Autodesk Inventor part; units mm, degrees
ref_plane "YZ Plane" through (0, 0, 0) normal (1, 0, 0) x (0, 1, 0)
ref_plane "XZ Plane" through (0, 0, 0) normal (0, 1, 0) x (-1, 0, 0)
ref_plane "XY Plane" through (0, 0, 0) normal (0, 0, 1) x (1, 0, 0)
sketch "Sketch1" plane through (0, 0, 0) normal (0, 1, 0) x (-1, 0, 0)
  line L0 (-60, 105) -> (60, 105)
  line L1 (60, 105) -> (60, 90)
  line L2 (60, -105) -> (-60, -105)
  line L3 (-60, -105) -> (-60, -90)
  line L4 (-60, 105) -> (60, -105) construction
  line L5 (60, 105) -> (-60, -105) construction
  line L6 (60, 90) -> (-60, 90)
  line L7 (60, -90) -> (-60, -90)
  line L8 (60, 90) -> (60, -90)
  line L9 (60, -90) -> (60, -105)
  line L10 (-60, -90) -> (-60, 90)
  line L11 (-60, 90) -> (-60, 105)
  line L12 (84, 0) -> (-84, 0)
  line L13 (0, -147) -> (0, 147)
  point P0 (0, 0)
  dimension "d0" = 180
  dimension "d1" = 15
  dimension "d2" = 120
extrude "Plate1" add sketch "Sketch1" along normal blind 5 contours L6 L13 L12 L10 | L6 L8 L12 L13 | L12 L13 L7 L10 | L12 L8 L7 L13
sketch "Sketch2" plane through (-60, 5, 85) normal (0, 0, 1) x (1, 0, 0)
  line L0 (120, 0) -> (0, 0)
  line L1 (0, 0) -> (0, -15)
  line L2 (0, -15) -> (120, -15)
  line L3 (120, -15) -> (120, 0)
edge flange "Flange1" height 15 angle 90 thickness 5 bend radius 5 thickness toward (0, 0, 1) relief tear relief width 5 relief depth 2.5 corner gap 5 corner form 0 edges at (0, 0, 90) (0, 0, -90) wall of the first edge with corners at (60, 5, 85) (-60, 5, 85) (-60, -10, 85) (60, -10, 85)
bend "Bend1"
corner "Corner1"
sketch "Sketch3" plane through (0, 0, 0) normal (0, -1, 0) x (1, 0, 0)
  circle A0 centre (-16.2613, 28.9263) radius 2.75
  circle A1 centre (38.7387, 28.9263) radius 2.75
  circle A2 centre (-16.2613, -31.0737) radius 2.75
  circle A3 centre (38.7387, -31.0737) radius 2.75
  point P0 (0, 0)
extrude "Extrusion1" cut sketch "Sketch3" against normal through all
equation "\"d3\" = Thickness"
equation "\"d4\" = BendReliefWidth"
equation "\"d5\" = BendReliefDepth"
equation "\"d6\" = MinimumRemnant"
equation "\"d7\" = TransitionRadius"
equation "\"d10\" = BendRadius"
equation "\"d11\" = CornerReliefSize"
equation "\"d12\" = GapSize"
equation "\"d13\" = JacobiRadiusSize"
equation "\"BendRadius\" = Thickness"
equation "\"BendReliefWidth\" = Thickness"
equation "\"BendReliefDepth\" = 0.5 * Thickness"
equation "\"TransitionRadius\" = BendRadius"
equation "\"JacobiRadiusSize\" = BendRadius"
equation "\"GapSize\" = Thickness"
properties part number "shapeoko_zplate"
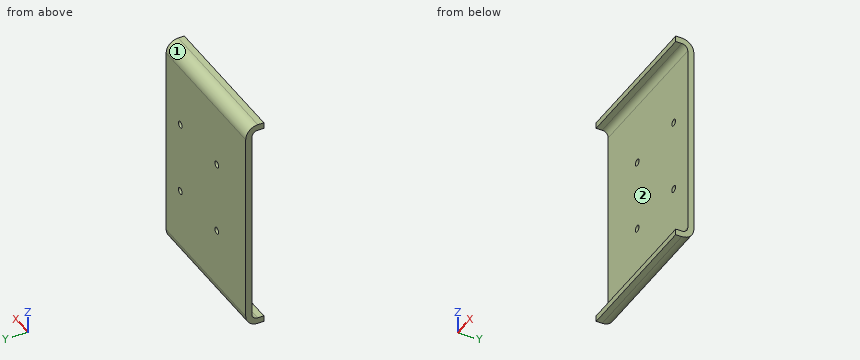
Design review of the part built by this model. Coordinates are the model's own, in mm. Face numbers are marked on the shaded views. A direction names the side the tool comes from. Round coordinates to 2 decimals unless told otherwise and drop trailing zeros. Write each loop counter-clockwise with the first axis right and the second up, starting at its lowest first coordinate (ties: lowest second). Pieces come first, ordered by that corner, then holes. Notation, with made-up numbers: (18.25, 32.5) -> (64.25, 32.5) arc R18 ccw to (64.25, 46.5) -> close; hole circle Ø4 at (31.25, 67). An arc over 180 degrees is marked (long way). Answer in a Markdown table with one row per item.
Q1. Take a section at D-D, the plane x = 39.5. State the section outline as (y, z) points.
The answers:
| item | result |
|---|---|
| outline | (-10, -90) -> (-5, -90) arc R10 ccw to (5, -80) -> (5, -33.72) -> (0, -33.72) -> (0, -80) arc R5 cw to (-5, -85) -> (-10, -85) -> close; (-10, 85) -> (-5, 85) arc R5 cw to (0, 80) -> (0, 31.57) -> (5, 31.57) -> (5, 80) arc R10 ccw to (-5, 90) -> (-10, 90) -> close; (0, -28.43) -> (5, -28.43) -> (5, 26.28) -> (0, 26.28) -> close |
Q2. To check wall thickness, follow L1, parallel to Z at x = -14, y = 3.75; L2, parallel to Z at x = -49.5, y = -4.5; L3, parallel to Y at x = 32, z = 25. State the ranges of each line that lie inside material, in increasing order. Write a range as [from, to].
The answers:
| item | result |
|---|---|
| L1 | [-84.84, -32.64], [-29.51, 27.36], [30.49, 84.84] |
| L2 | [-89.99, -84.97], [84.97, 89.99] |
| L3 | [0, 5] |
Q3. Take a section at A-A, the plane y = -7.5. State the section outline as (x, z) points.
The answers:
| item | result |
|---|---|
| outline | (-60, -90) -> (60, -90) -> (60, -85) -> (-60, -85) -> close; (-60, 85) -> (60, 85) -> (60, 90) -> (-60, 90) -> close |
Q4. Take a section at B-B, the plane x = -43.5. State the section outline as (y, z) points, then the cut area to 3 significant figures.
The answers:
| item | result |
|---|---|
| outline | (-10, -90) -> (-5, -90) arc R10 ccw to (5, -80) -> (5, 80) arc R10 ccw to (-5, 90) -> (-10, 90) -> (-10, 85) -> (-5, 85) arc R5 cw to (0, 80) -> (0, -80) arc R5 cw to (-5, -85) -> (-10, -85) -> close |
| area | 968 mm² |
Q5. For the marked faces 1 and 2, list the 3-axis set-ups (+Z, -Z, +X, -X, +Y, -Y) from which the entire face can be reached by the end or side of a thin tool; tool diameter is ignored.
The answers:
| item | result |
|---|---|
| face 1 | +Z, +X, -X, +Y |
| face 2 | +X, -X, -Y |
Q6. Take a section at C-C, the plane y = 3.25. State the section outline as (x, z) points.
The answers:
| item | result |
|---|---|
| outline | (-60, -85.65) -> (60, -85.65) -> (60, 85.65) -> (-60, 85.65) -> close; hole circle Ø5.5 at (-16.26, -31.07); hole circle Ø5.5 at (-16.26, 28.93); hole circle Ø5.5 at (38.74, -31.07); hole circle Ø5.5 at (38.74, 28.93) |
Q7. Clearance check with flat-ended pins moving along their axes: pin 1 Ø9 at (x, z) = (-16.26, 28.93) entering from -Y; pin 2 Ø5 at (x, z) = (-16.26, -31.07) entering from -Y. State where each tip first meets the part, or that it passes through.
The answers:
| item | result |
|---|---|
| pin 1 | y = 0 |
| pin 2 | through |
